Part model, mm, in its own coordinate system. A direction names the side the tool comes from. Coordinates: 2 decimals unless noted, no trailing zeros. Order: outer loops, then holes, each group sorted by start corner. A loop starts at its lowest first (then second) coordinate and runs counter-clockwise, first axis right, second up.
```python
from build123d import *

# Parameters (mm, degrees)
BOSS_EXTRUDE1_DEPTH = 13.3
SKETCH1_3_R         = 1.5
BOSS_EXTRUDE2_DEPTH = 2
SKETCH2_W           = 29.2
SKETCH2_H           = 10
BOSS_EXTRUDE3_DEPTH = 16.3


with BuildPart() as part:
    # Sketch1 → Boss-Extrude1 (new body)
    with BuildSketch(Plane(origin=(0, 0, 0), x_dir=(1, 0, 0), z_dir=(0, 1, 0))):
        Polygon((-24.5, -16.7), (-2.5, -16.7), (2.5, -16.7), (24.5, -16.7), (24.5, 16.7), (2.5, 16.7), (-2.5, 16.7), (-24.5, 16.7), align=None)
    extrude(amount=BOSS_EXTRUDE1_DEPTH)

    # Sketch1_3 → Boss-Extrude2 (add)
    # profile 1 of 2: a face of its own
    with BuildSketch(Plane(origin=(0, 0, 0), x_dir=(1, 0, 0), z_dir=(0, 1, 0))):
        with BuildLine():
            Line((-2.5, -20), (-2.5, -16.7))
            Line((-2.5, -16.7), (2.5, -16.7))
            Line((2.5, -16.7), (2.5, -20))
            ThreePointArc((2.5, -20), (0, -22.5), (-2.5, -20))
        make_face()
        with Locations(Location((0, -20, 0), (0, 0, 270))):
            Circle(SKETCH1_3_R, mode=Mode.SUBTRACT)
    # profile 2 of 2: a face of its own
    with BuildSketch(Plane(origin=(0, 0, 0), x_dir=(1, 0, 0), z_dir=(0, 1, 0))):
        with BuildLine():
            Line((2.5, 20), (2.5, 16.7))
            Line((2.5, 16.7), (-2.5, 16.7))
            Line((-2.5, 16.7), (-2.5, 20))
            ThreePointArc((-2.5, 20), (0, 22.5), (2.5, 20))
        make_face()
        with Locations(Location((0, 20, 0), (0, 0, 270))):
            Circle(SKETCH1_3_R, mode=Mode.SUBTRACT)
    extrude(amount=BOSS_EXTRUDE2_DEPTH)

    # Sketch2 → Boss-Extrude3 (add)
    with BuildSketch(Plane(origin=(0, 0, 0), x_dir=(1, 0, 0), z_dir=(0, 1, 0))):
        with Locations((-9.9, 11.7)):
            Rectangle(SKETCH2_W, SKETCH2_H)
    extrude(amount=BOSS_EXTRUDE3_DEPTH)


solid = part.part
```
(1) Drop flat-ended pins along their axis: pin 1 (4 mm diameter, centred on x = 0, z = 18.5, fed in from +Y); pin 2 (2 mm diameter, centred on y = 1, z = -19, fed in from -X); pin 3 (2 mm diameter, centred on y = 1, z = 18.5, fed in from +X). Give the stop position or say it passes through.
(2) Slice it at C-C, the plane z = -15. Give the cut face in (x, y).
(3) Probe line 1 (X direction, y = 0.4, z = 20); line 2 (Y direction, x = 22.5, z = 1.5); line 3 (Z direction, x = -19.5, y = 4.5). List the from-to ranges inside material, lowest first.
(4) Slice it at A-A, the plane x = 0. Give the cut face in (y, z), then the cut area to 3 significant figures.
(5) Slice it at D-D, the plane x = -20. Give the cut face in (y, z).
(6) Tool access for faces 1 (the face through (4.7, 15, -12)), 2 (the face through (-2.5, 1, -18)), 3 (the face through (0, 2, -18)), 4 (the face through (0, 2, 18)), 5 (the face through (2.5, 1, 18)): list every direction of +Z, -Z, +X, -X, +Y, -Y with a clear straight run to the whole face (end or side of a thin tool).
(7) Slice it at B-B, the plane y = 6. Give the cut face in (x, z).
Here are the results:
1. pin 1: stops at y = 13.3
1. pin 2: stops at x = -2.5
1. pin 3: stops at x = 2.5
2. outline: (-24.5, 0) - (24.5, 0) - (24.5, 13.3) - (4.7, 13.3) - (4.7, 16.3) - (-24.5, 16.3) - close
3. line 1: x = -2.5 to -1.5, 1.5 to 2.5
3. line 2: y = 0 to 13.3
3. line 3: z = -16.7 to 16.7
4. outline: (0, -22.5) - (2, -22.5) - (2, -21.5) - (0, -21.5) - close; (0, -18.5) - (2, -18.5) - (2, -16.7) - (16.3, -16.7) - (16.3, -6.7) - (13.3, -6.7) - (13.3, 16.7) - (2, 16.7) - (2, 18.5) - (0, 18.5) - close; (0, 21.5) - (2, 21.5) - (2, 22.5) - (0, 22.5) - close
4. area: 485 mm2
5. outline: (0, -16.7) - (16.3, -16.7) - (16.3, -6.7) - (13.3, -6.7) - (13.3, 16.7) - (0, 16.7) - close
6. face 1: +Z, -Z, +X, +Y
6. face 2: -Z, -X, +Y, -Y
6. face 3: -Z, +X, -X, +Y
6. face 4: +Z, +X, -X, +Y
6. face 5: +Z, +X, +Y, -Y
7. outline: (-24.5, -16.7) - (24.5, -16.7) - (24.5, 16.7) - (-24.5, 16.7) - close
